Build history of the part. All positions in model axes, mm. Give positions to 0.01 mm unless a question says otherwise; leave off trailing zeros. Write each loop counter-clockwise with the first axis right and the second up, starting at its lowest first coordinate (ties: lowest second). Pieces come first, ordered by that corner, then holes.
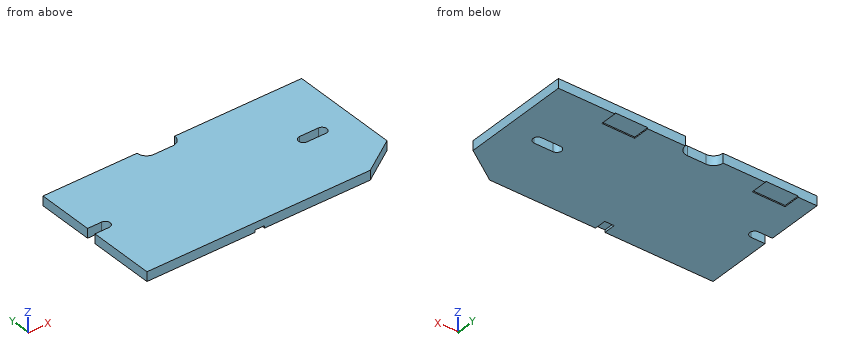
from build123d import *

# Parameters (mm, degrees)
F0_W      = 698.5
F0_H      = 355.6
F1_DEPTH  = 25.4
F3_DEPTH  = 25.401
F4_W      = 88.9
F4_H      = 44.45
F5_DEPTH  = 3.175
F7_DEPTH  = 25.401
F8_W      = 101.6
F8_H      = 25.4
F9_DEPTH  = 25.4
F10_R     = 25.39999
F11_W     = 25.4
F11_H     = 31.75
F12_DEPTH = 6.35


# Not quite as in the source:
# - a fillet or chamfer is up to 0.001 mm smaller than in the source, because OpenCascade refuses the exact size
# - a feature names something its author has since deleted; it is built from what else it names


with BuildPart() as f1:
    # F0 (on Top) → F1 (new body)
    with BuildSketch(Plane.XY):
        Rectangle(F0_W, F0_H)
    extrude(amount=F1_DEPTH)

    # F2 (on face) → F3 (cut, through all)
    with BuildSketch(Plane.XY.offset(25.4)):
        Polygon((349.25, -114.3), (254, -177.8), (349.25, -177.8), align=None)
    extrude(amount=-F3_DEPTH, mode=Mode.SUBTRACT)

    # F4 (on face) → F5 (cut)
    with BuildSketch(Plane(origin=(0, 0, 0), x_dir=(1, 0, 0), z_dir=(0, 0, -1))):
        with Locations((-254, -155.575)):
            Rectangle(F4_W, F4_H)
        with Locations((152.4, -155.575)):
            Rectangle(F4_W, F4_H)
    extrude(amount=-F5_DEPTH, mode=Mode.SUBTRACT)

    # F6 (on face) → F7 (cut, through all)
    with BuildSketch(Plane.XY.offset(25.4)):
        with BuildLine():
            Line((-311.747228622, 0), (-311.747228622, 0.0140503716))
            ThreePointArc((-311.747228622, 0.0140503716), (-298.45, 12.7), (-311.747228622, 25.3859496284))
            Line((-311.747228622, 25.3859496284), (-382.2402954102, 25.3859496284))
            Line((-382.2402954102, 25.3859496284), (-382.2402954102, 0))
            Line((-382.2402954102, 0), (-311.747228622, 0))
        make_face()
        with BuildLine():
            Line((264.16, 12.6990057829), (213.5189091712, 12.6990057829))
            ThreePointArc((213.5189091712, 12.6990057829), (200.66, 0), (213.5189091712, -12.6990057829))
            Line((213.5189091712, -12.6990057829), (213.5189091712, -12.7009942171))
            Line((213.5189091712, -12.7009942171), (264.16, -12.7009942171))
            ThreePointArc((264.16, -12.7009942171), (276.86, -0.0009942171), (264.16, 12.6990057829))
        make_face()
    extrude(amount=-F7_DEPTH, mode=Mode.SUBTRACT)

    # F8 (on face) → F9 (cut)
    with BuildSketch(Plane.XY.offset(25.4)):
        with Locations((-44.45, 165.1)):
            Rectangle(F8_W, F8_H)
    extrude(amount=-F9_DEPTH, mode=Mode.SUBTRACT)

    # F10 (radius 25.4 in the source; OpenCascade refuses exactly that, so slightly less here)
    f10_edges = [f1.edges().sort_by_distance(p)[0] for p in [
        (-95.25, 152.4, 12.7),
        (6.35, 152.4, 12.7),
    ]]
    fillet(f10_edges, radius=F10_R)

    # F11 (on face) → F12 (cut)
    with BuildSketch(Plane(origin=(0, 0, 0), x_dir=(1, 0, 0), z_dir=(0, 0, -1))):
        with Locations((-44.45, 161.925)):
            Rectangle(F11_W, F11_H)
    extrude(amount=-F12_DEPTH, mode=Mode.SUBTRACT)


solid = f1.part
(1) Saw through at C-C, the plane x = -4.5. List the corners of the cut face in (y, z).
(2) Saw through at B-B, the plane x = 306.5. List the corners of the cut face in (y, z), plus the area to 3 significant figures.
(3) Probe line 1 (Y direction, x = 243.5, z = 21.75); line 2 (Z direction, x = 193.5, y = 147) (3 decimals); line 3 (Y direction, x = -82.5, z = 16.5). List the from-to ranges inside material, lowest first.
(4) Drop flat-ended pins along their axis: pin 1 (1 mm diameter, centred on x = 155.5, z = 1.5, fed in from +Y); pin 2 (7.5 mm diameter, centred on x = -47, y = -160.5, fed in from -Z); pin 3 (12 mm diameter, centred on y = -126.5, z = 19.5, fed in from +X). Give the stop position or say it passes through.
Computed values:
1. outline: (-177.8, 0) - (156.98, 0) - (156.98, 25.4) - (-177.8, 25.4) - close
2. outline: (-142.8, 0) - (177.8, 0) - (177.8, 25.4) - (-142.8, 25.4) - close
2. area: 8,140 mm2
3. line 1: y = -177.8 to -12.7, 12.7 to 177.8
3. line 2: z = 3.175 to 25.4
3. line 3: y = -177.8 to 155.77
4. pin 1: stops at y = 133.35
4. pin 2: stops at z = 6.35
4. pin 3: stops at x = 339.95
